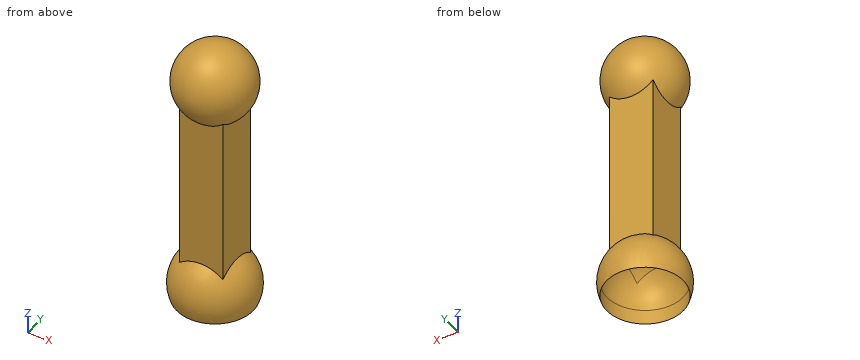
from build123d import *
from build123d import SkipClean  # not in build123d's __all__

# Parameters (mm, degrees)
F2_W     = 8
F2_H     = 8
F3_DEPTH = 40
F4_R     = 7
F5_DEPTH = 7.5
F6_W     = 4
F6_H     = 8
F8_W     = 4
F8_H     = 8


# Not quite as in the source:
# - a feature names something its author has since deleted; it is built from what else it names


with BuildPart() as f1:
    # F0 (on Top) → F1 (revolve)
    with BuildSketch(Plane.XY):
        with BuildLine():
            Line((7, 0), (7.5, 0))
            ThreePointArc((7.5, 0), (0, 7.5), (-7.5, 0))
            Line((-7.5, 0), (-7, 0))
            ThreePointArc((-7, 0), (0, 7), (7, 0))
        make_face()
    revolve(axis=Axis((0, 0, 0), (-1, 0, 0)))

    # F2 (on Top) → F3 (join)
    with BuildSketch(Plane.XY):
        Rectangle(F2_W, F2_H)
    extrude(amount=F3_DEPTH)

    # F4 (on Top) → F5 (cut)
    with BuildSketch(Plane.XY):
        Circle(F4_R)
    extrude(amount=-F5_DEPTH, mode=Mode.SUBTRACT)

    # F6 (on face) → F7 (revolve, cut)
    with BuildSketch(Plane(origin=(0, 0, 0), x_dir=(1, 0, 0), z_dir=(0, 0, -1))):
        with BuildLine():
            ThreePointArc((0, -7), (7, 0), (0, 7))
            Line((0, 7), (0, 4))
            Line((0, 4), (4, 4))
            Line((4, 4), (4, -4))
            Line((4, -4), (0, -4))
            Line((0, -4), (0, -7))
        make_face()
        with Locations((2, 0)):
            Rectangle(F6_W, F6_H)
    with SkipClean():  # cleaning this boolean's faces spoils the solid; the shape is the same uncleaned
        revolve(axis=Axis((0, 0, 0), (0, 1, 0)), mode=Mode.SUBTRACT)

    # F8 (on face) → F9 (revolve)
    with BuildSketch(Plane.XY.offset(40)):
        with BuildLine():
            ThreePointArc((0, -7), (7, 0), (0, 7))
            Line((0, 7), (0, 4))
            Line((0, 4), (4, 4))
            Line((4, 4), (4, -4))
            Line((4, -4), (0, -4))
            Line((0, -4), (0, -7))
        make_face()
        with Locations((2, 0)):
            Rectangle(F8_W, F8_H)
    with SkipClean():  # cleaning this boolean's faces spoils the solid; the shape is the same uncleaned
        revolve(axis=Axis((0, 0, 40), (0, -1, 0)))


solid = f1.part
Can you work these out from the model? Positions are in its coordinate system, mm. Give positions to 0.01 mm unless a question says otherwise; leave off trailing zeros. Loops run counter-clockwise (first coordinate to the right, second up) from the corner with the lowest first, then second, coordinate; pieces in that order, holes last. Notation, with made-up numbers: M -18.5,76.5 L 34.5,76.5 A12 cw 34.5,84.5 Z; hole C -4,-39 d6. An arc over 180 degrees is marked long. One line per item, written item: value.
1) Please list where these lines run through material, in increasing order: line 1 (X direction, y = 1, z = 18); line 2 (X direction, y = 0, z = -1.7).
Geometry check:
line 1: x = -4 to 4
line 2: x = -7.3 to -7, 7 to 7.3
2) Imagine slicing it at B-B on y = 0.75. Write out the boundary of the cut face in (x, z), and give its area (3 significant figures).
Geometry check:
outline: M -6.96,-2.69 L -6.96,0 A6.96 cw 6.96,0 L 6.96,-2.69 A7.46 ccw 4,6.3 L 4,34.3 A6.96 ccw long -4,34.3 L -4,6.3 A7.46 ccw Z
area: 376 mm²
3) Imagine slicing it at C-C on x = 5.75. Write out the boundary of the cut face in (y, z), and give its area (3 significant figures).
Geometry check:
outline: M -3.99,-2.69 L -3.99,0 A3.99 cw 3.99,0 L 3.99,-2.69 A4.82 ccw long Z; C 0,40 d7.98
area: 64.5 mm²
4) I'm going to push flat-ended pins straight in: pin 1 (6.5 mm diameter, centred on y = 0.5, z = 19.5, fed in from +X); pin 2 (6.5 mm diameter, centred on y = -1.5, z = 17.5, fed in from -X); pin 3 (4 mm diameter, centred on x = 1.5, z = 21.5, fed in from +Y). Where does each tip first touch, or does it pass through?
Geometry check:
pin 1: stops at x = 4
pin 2: stops at x = -4
pin 3: stops at y = 4
5) Imagine slicing it at A-A on x = 2.5. Write out the boundary of the cut face in (y, z), and give its area (3 significant figures).
Geometry check:
outline: M -6.54,-2.69 L -6.54,0 A6.54 cw 6.54,0 L 6.54,-2.69 A7.07 ccw 4,5.83 L 4,34.83 A6.54 ccw long -4,34.83 L -4,5.83 A7.07 ccw Z
area: 365 mm²
